Design review of the part built by this model. Coordinates are the model's own, in mm. A direction names the side the tool comes from. Coordinates: 2 decimals unless noted, no trailing zeros. Write each loop counter-clockwise with the first axis right and the second up, starting at its lowest first coordinate (ties: lowest second). Pieces come first, ordered by that corner, then holes.
Q1. The part is to be moulded in two halves that separate along X. For faces 1 (the face through (-24.538, -25.496, -2.447)), 2 (the face through (-21.8, -21.6, -4.826)), 3 (the face through (-28.547, 1.256, -27.491)), say which applies: +X half, -X half, draft (parallel to the pull), parting line (faces both ways), or undercut.
Q2. Add section A-A, the plane y = 23.5. Give the boundary of the cut face in (x, z) (3 decimals).
Q3. Add section C-C, the plane z = -19. Give the boundary of the cut face in (x, y) (3 decimals), plus the area to 3 significant figures.
Q4. Machinability: for faces 4 (the face through (21.6, -21.6, -4.826)), 5 (the face through (-0.4, 19.5, 0)), 6 (the face through (28.575, 0, -2)), 7 (the face through (-21.8, 21.8, -4.826)), 8 (the face through (21.6, 21.8, -4.826)), which of the approach directions +Z, -Z, +X, -X, +Y, -Y give a long, thin tool a straight path to every point of the face, cutting with its end or side? Answer none if there is none.
Q5. Clearance check with flat-ended pins moving along their axes: pin 1 Ø5 at (x, y) = (-23.5, 23.5) entering from -Z; pin 2 Ø6 at (x, y) = (-23.5, -23.5) entering from +Z; pin 3 Ø1 at (y, z) = (-20.5, -41) entering from -X; pin 4 Ø2.5 at (x, y) = (23.5, -23.5) entering from -Z. State where each tip first meets the part, or that it passes through.
Q6. Add section B-B, the plane x = 7. Give the boundary of the cut face in (y, z) (3 decimals).
Q7. To check wall thickness, follow probe 1 along Y at (x, z) = (23.5, -1.25) (3 decimals); probe 2 along X at (y, z) = (-23, -2) (3 decimals); probe 3 along Z at (x, y) = (-6.5, -2). State the ranges of each line that lie inside material, in increasing order.
from build123d import *

# Parameters (mm, degrees)
SKETCH1_W            = 57.15
SKETCH1_H            = 57.15
BOSS_EXTRUDE1_DEPTH  = 4.826
SKETCH2_R            = 19.05
BOSS_EXTRUDE2_DEPTH  = 1.524
SKETCH3_R            = 3.175
BOSS_EXTRUDE3_DEPTH  = 20.574
SKETCH5_R            = 28.575
BOSS_EXTRUDE4_DEPTH  = 50.8
M4_CLEARANCE_HOLE1_D = 4.5
FILLET1_R            = 3.175


with BuildPart() as part:
    # Sketch1 → Boss-Extrude1 (new body)
    with BuildSketch(Plane.XY):
        Rectangle(SKETCH1_W, SKETCH1_H)
    extrude(amount=-BOSS_EXTRUDE1_DEPTH)

    # Sketch2 → Boss-Extrude2 (add)
    with BuildSketch(Plane.XY):
        with Locations(Location((0, 0, 0), (0, 0, 180))):
            Circle(SKETCH2_R)
    extrude(amount=BOSS_EXTRUDE2_DEPTH)

    # Sketch3 → Boss-Extrude3 (add)
    with BuildSketch(Plane.XY):
        Circle(SKETCH3_R)
    extrude(amount=BOSS_EXTRUDE3_DEPTH)

    # Sketch5 → Boss-Extrude4 (add)
    with BuildSketch(Plane.XY):
        Circle(SKETCH5_R)
    extrude(amount=-BOSS_EXTRUDE4_DEPTH)

    # M4 Clearance Hole1 (through all)
    with Locations(Plane.XY):
        with Locations((-23.5, 23.5), (23.5, 23.5), (23.5, -23.5), (-23.5, -23.5)):
            Hole(M4_CLEARANCE_HOLE1_D / 2)

    # Fillet1
    fillet1_edges = [part.edges().sort_by_distance(p)[0] for p in [
        (28.575, -28.575, -2.413),
        (-28.575, -28.575, -2.413),
        (-28.575, 28.575, -2.413),
        (28.575, 28.575, -2.413),
    ]]
    fillet(fillet1_edges, radius=FILLET1_R)


solid = part.part
Here are the results:
1. face 1: undercut
1. face 2: draft
1. face 3: parting line
2. outline: (-28.575, -4.826) - (-25.75, -4.826) - (-25.75, 0) - (-28.575, 0) - close; (-21.25, -4.826) - (-16.257, -4.826) - (-16.257, -50.8) - (16.257, -50.8) - (16.257, -4.826) - (21.25, -4.826) - (21.25, 0) - (-21.25, 0) - close; (25.75, -4.826) - (28.575, -4.826) - (28.575, 0) - (25.75, 0) - close
3. outline: circle Ø57.15 at (0, 0)
3. area: 2,570 mm2
4. face 4: -Z, +X, -Y
4. face 5: +Z
4. face 6: +Z, -Z, +X, +Y, -Y
4. face 7: -Z, -X, +Y
4. face 8: -Z, +X, +Y
5. pin 1: stops at z = -4.83
5. pin 2: stops at z = 0
5. pin 3: stops at x = -20.41
5. pin 4: passes through
6. outline: (-28.575, -4.826) - (-27.704, -4.826) - (-27.704, -50.8) - (27.704, -50.8) - (27.704, -4.826) - (28.575, -4.826) - (28.575, 0) - (17.717, 0) - (17.717, 1.524) - (-17.717, 1.524) - (-17.717, 0) - (-28.575, 0) - close
7. probe 1: y = -28.575 to -25.75, -21.25 to 21.25, 25.75 to 28.575
7. probe 2: x = -28.575 to -25.694, -21.306 to 21.306, 25.694 to 28.575
7. probe 3: z = -50.8 to 1.52
